Study the drawing (mm; zero at the part's minimum x, y, z) and answer. Round coordinates to 2 decimals unless told otherwise and drop trailing zeros. Order: outer loops, then holes, each group sorted by start corner. A loop starts at its lowest first (then second) coordinate and runs counter-clockwise, first axis right, second up. Notation, with made-up numbers: (33, 38) - (50, 38) arc R25 cw to (50, 52) - close; hole circle Ø5 at (69, 29.25). An arc over 180 degrees is marked (long way). Put each result on its own line as item: value.
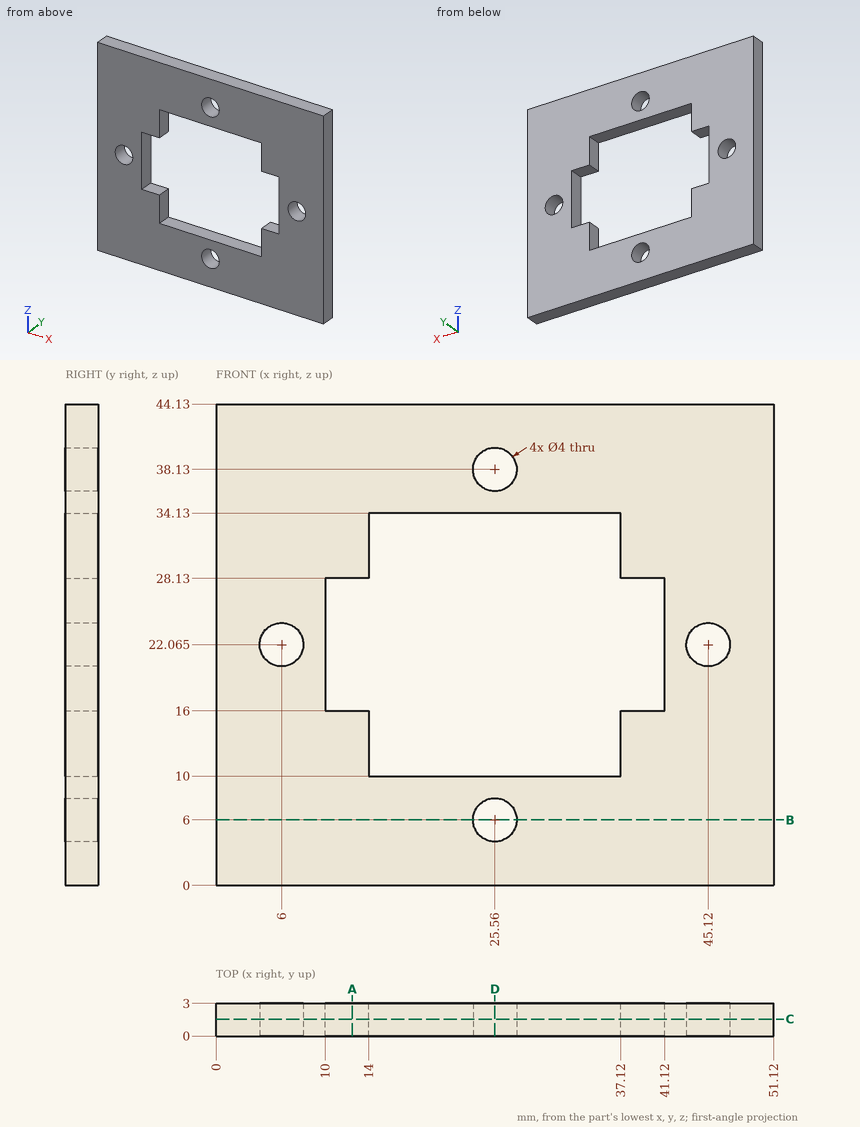
1) A cutting plane is placed at C-C on y = 1.55. Write down the section's boundary in (x, z) (3 decimals).
Findings below:
outline: (0, 0) - (51.12, 0) - (51.12, 44.13) - (0, 44.13) - close; hole circle Ø4 at (6, 22.065); hole (10, 16) - (14, 16) - (14, 10) - (37.12, 10) - (37.12, 16) - (41.12, 16) - (41.12, 28.13) - (37.12, 28.13) - (37.12, 34.13) - (14, 34.13) - (14, 28.13) - (10, 28.13) - close; hole circle Ø4 at (25.56, 6); hole circle Ø4 at (25.56, 38.13); hole circle Ø4 at (45.12, 22.065)
2) A cutting plane is placed at A-A on x = 12.5. Write down the section's boundary in (y, z).
Findings below:
outline: (0, 0) - (3, 0) - (3, 16) - (0, 16) - close; (0, 28.13) - (3, 28.13) - (3, 44.13) - (0, 44.13) - close
3) A cutting plane is placed at D-D on x = 25.56. Write down the section's boundary in (y, z).
Findings below:
outline: (0, 0) - (3, 0) - (3, 4) - (0, 4) - close; (0, 8) - (3, 8) - (3, 10) - (0, 10) - close; (0, 34.13) - (3, 34.13) - (3, 36.13) - (0, 36.13) - close; (0, 40.13) - (3, 40.13) - (3, 44.13) - (0, 44.13) - close
4) A cutting plane is placed at B-B on z = 6. Write down the section's boundary in (x, y).
Findings below:
outline: (0, 0) - (23.56, 0) - (23.56, 3) - (0, 3) - close; (27.56, 0) - (51.12, 0) - (51.12, 3) - (27.56, 3) - close
5) Given pin 1 Ø3.5 at (x, z) = (25.56, 38.13) entering from +Y, flat-ended and moving along its own axis, determine where the tip first touches the part or whether it passes through.
Findings below:
pin 1: passes through
6) Straight lines are drawn through the part: L1, parallel to X at y = 2.5, z = 15; L2, parallel to X at y = 0.95, z = 26.5; L3, parallel to X at y = 1.3, z = 23. For each, find the intervals that lie inside material, in ascending order. Write a range as from..to.
Findings below:
L1: x = 0..14, 37.12..51.12
L2: x = 0..10, 41.12..51.12
L3: x = 0..4.23, 7.77..10, 41.12..43.35, 46.89..51.12
